The figure shows three views and two pictorial views of one solid part (mm, origin at its lowest corner). Answer the questions. A direction names the side the tool comes from. Give positions to 0.01 mm unless a question says otherwise; leave off trailing zeros. Order: outer loops, then holes, each group sorted by start corner. A loop starts at its lowest first (then second) coordinate and runs counter-clockwise, first axis right, second up. Notation, with made-up numbers: (81, 55) -> (112, 55) arc R21 ccw to (112, 85) -> close; hole circle Ø5 at (30, -38). An arc over 180 degrees is marked (long way). Use one line per item in the form item = value.
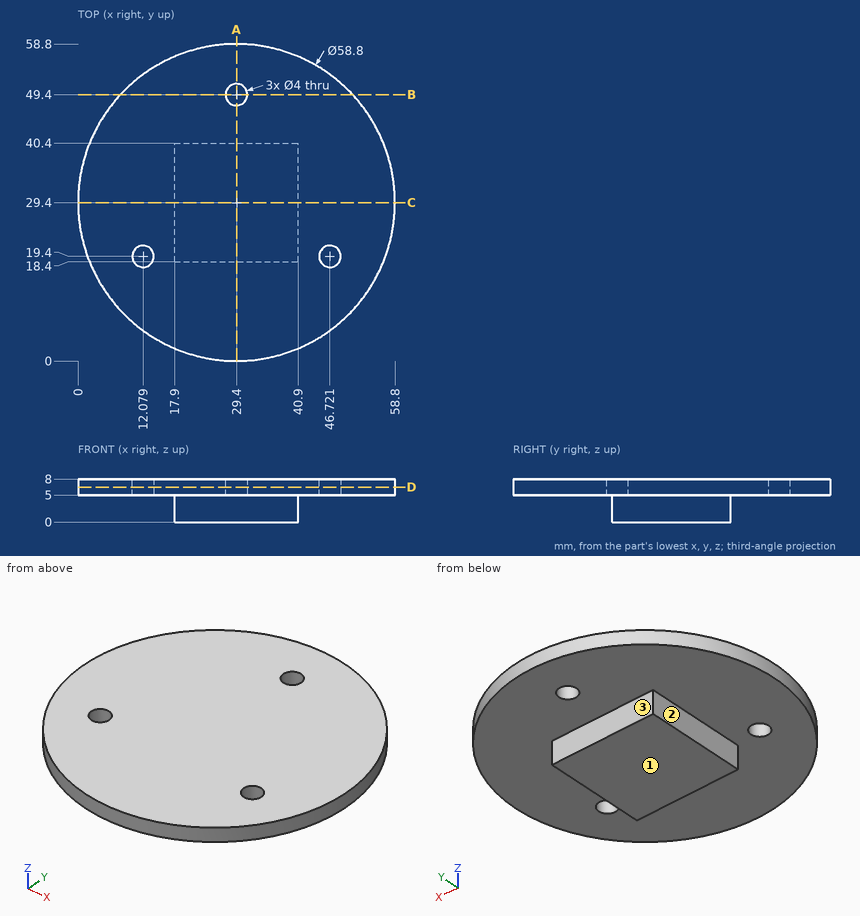
Item 1: The part is cut by section C-C on y = 29.4. Give the vertices of the cut face in (x, z).
Checks:
outline = (0, 5) -> (17.9, 5) -> (17.9, 0) -> (40.9, 0) -> (40.9, 5) -> (58.8, 5) -> (58.8, 8) -> (0, 8) -> close
Item 2: Given pin 1 Ø3 at (y, z) = (49, 5) entering from -X; pin 2 Ø2 at (y, z) = (24.5, 2.5) entering from +X; pin 3 Ø4 at (x, z) = (28, 7) entering from -Y; pin 4 Ø2.5 at (x, y) = (29.4, 49.4) entering from +Z, each flat-ended and moving along its own axis, determine where each tip first touches the part or whether it passes through.
Checks:
pin_1 = 6.23
pin_2 = 40.9
pin_3 = 0
pin_4 = through
Item 3: Straight lines are drawn through the part: L1, parallel to Y at x = 29.4, z = 6.35; L2, parallel to Z at x = 43, y = 29.5; L3, parallel to Y at x = 27.5, z = 4. For each, find the intervals that lie inside material, in ascending order. Write a range as from..to.
Checks:
L1 = 0..47.4, 51.4..58.8
L2 = 5..8
L3 = 18.4..40.4
Item 4: Which of the six approach directions +Z, -Z, +X, -X, +Y, -Y give full straight-line access (tool end or side, diameter ignored) to the marked faces 1, 2 and 3?
Checks:
face_1 = -Z, +X, -X, +Y, -Y
face_2 = -Z, -X, +Y, -Y
face_3 = -Z, +X, -X, +Y
Item 5: The part is cut by section B-B on y = 49.4. Give the vertices of the cut face in (x, z).
Checks:
outline = (7.85, 5) -> (27.4, 5) -> (27.4, 8) -> (7.85, 8) -> close; (31.4, 5) -> (50.95, 5) -> (50.95, 8) -> (31.4, 8) -> close
Item 6: The part is cut by section D-D on z = 6.5. Give the vertices of the cut face in (x, y), and give its area (3 significant figures).
Checks:
outline = circle Ø58.8 at (29.4, 29.4); hole circle Ø4 at (12.08, 19.4); hole circle Ø4 at (29.4, 49.4); hole circle Ø4 at (46.72, 19.4)
area = 2,680 mm²
Item 7: The part is cut by section A-A on x = 29.4. Give the vertices of the cut face in (y, z).
Checks:
outline = (0, 5) -> (18.4, 5) -> (18.4, 0) -> (40.4, 0) -> (40.4, 5) -> (47.4, 5) -> (47.4, 8) -> (0, 8) -> close; (51.4, 5) -> (58.8, 5) -> (58.8, 8) -> (51.4, 8) -> close
